Model file for the job. Use its own axes, mm. A direction names the side the tool comes from. Give positions to 0.01 mm unless a question says otherwise; leave off trailing zeros. Order: outer loops, then holes, each group sorted by start corner. A loop starts at its lowest first (then second) coordinate and runs counter-clockwise, first axis right, second up. Notation, with made-up numbers: (14.5, 2.25) -> (55.5, 2.25) arc R12 cw to (55.5, 21.25) -> close; hole circle Ø11 at (33.5, 27.5). An arc over 180 degrees is marked (long way). Use CSV: the item, a comma, the result in double quotes. Start each with the question number.
1. 3-axis set-ups, long thin cutter, end or side, ignore diameter. For faces 5 (the flat face through (0, -18, 15)), 6 (the flat face through (0, -11, -13.675)), 7 (the flat face through (1, 3, 0)): which of +Z, -Z, +X, -X, +Y, -Y reach the whole face in a straight line?
2. Cut at A-A on x = -8.89. List the corners of the cut face in (y, z).
3. Wall check: line 1 (X direction, y = -20, z = -14) (3 decimals); line 2 (Z direction, x = -8.89, y = 1.25); line 3 (X direction, y = -10.5, z = -2) (3 decimals). Give the ranges that are in metal, low to high. Write a range as from..to.
4. Cut at D-D on z = 9.5. List the corners of the cut face in (x, y) (3 decimals), then the cut area to 3 significant figures.
5. Cut at B-B on y = -3.25. List the corners of the cut face in (x, z) (3 decimals), then the cut area to 3 significant figures.
6. Pull direction Z, two halves, no side cores. Call faces 1 (the cylindrical face through (20.85, 1.48, -1.83)), 2 (the flat face through (1, -10, -16.675)), 3 (the flat face through (-39.995, -10, 0)), 4 (the cylindrical face through (-38.85, -9.82, 14.07)): released by +Z, released by -Z, zero draft, split by the parting line, or undercut.
7. Cut at C-C on z = -1. List the corners of the cut face in (x, y) (1 decimal), then the cut area to 3 significant figures.
8. Drop flat-ended pins along their axis: pin 1 (0.9 mm diameter, centred on x = -6, z = 15.5, fed in from -Y); pin 2 (8 mm diameter, centred on x = 8, z = 5, fed in from -Y). Give the stop position or say it passes through.
Autodesk Inventor part; units mm, degrees
ref_plane "YZ Plane" through (0, 0, 0) normal (1, 0, 0) x (0, 1, 0)
ref_plane "XZ Plane" through (0, 0, 0) normal (0, 1, 0) x (-1, 0, 0)
ref_plane "XY Plane" through (0, 0, 0) normal (0, 0, 1) x (1, 0, 0)
sketch "Sketch1" plane through (0, 0, 0) normal (0, 1, 0) x (-1, 0, 0)
  line L0 (39.995, 16.6749) -> (-40.005, 16.6749)
  line L1 (-40.005, 16.6749) -> (-40.005, -16.6751)
  line L2 (-40.005, -16.6751) -> (39.995, -16.6751)
  line L3 (39.995, -16.6751) -> (39.995, 16.6749)
  circle A0 centre (-26.67, -0.0001) radius 6.1
  circle A1 centre (-8.89, -0.0001) radius 6.1
  circle A2 centre (8.89, -0.0001) radius 6.1
  circle A3 centre (26.67, -0.0001) radius 6.1
  point P0 (0, 0)
  dimension "d0" = 33.35
  dimension "d1" = 80
  dimension "d2" = 16.6751
  dimension "d3" = 40.005
  dimension "d4" = 12.2
  dimension "d5" = 13.335
  dimension "d8" = 17.78
extrude "Extrusion1" add sketch "Sketch1" along normal blind 3
sketch "Sketch2" plane through (0, 0, 0) normal (0, -1, 0) x (1, 0, 0)
  circle A0 centre (-26.67, -0.0001) radius 6.1
  circle A1 centre (-8.89, -0.0001) radius 6.1
  circle A2 centre (8.89, -0.0001) radius 6.1
  circle A3 centre (26.67, -0.0001) radius 6.1
  line L0 (-39.995, -16.6751) -> (-39.995, 16.6749)
  line L1 (-39.995, 16.6749) -> (40.005, 16.6749)
  line L2 (40.005, 16.6749) -> (40.005, -16.6751)
  line L3 (40.005, -16.6751) -> (-39.995, -16.6751)
  line L4 (33.899, -13.6749) -> (-33.899, -13.6749)
  line L5 (-33.899, -13.6749) -> (-33.899, 13.6749)
  line L6 (-33.899, 13.6749) -> (33.899, 13.6749)
  line L7 (33.899, 13.6749) -> (33.899, -13.6749)
  line L8 (33.899, -13.6749) -> (-33.899, 13.6749) construction
  line L9 (-33.899, -13.6749) -> (33.899, 13.6749) construction
  point P0 (0, 0)
  dimension "d15" = 6.096
  dimension "d16" = 6.106
  dimension "d17" = 3
  dimension "d18" = 7.229
extrude "Extrusion2" add sketch "Sketch2" along normal blind 23 contours L0 L1 L2 L3
sketch "Sketch4" plane through (-39.995, 3, 16.6749) normal (0, 0, 1) x (1, 0, 0)
  line L0 (80, -26) -> (0, -26)
  line L1 (0, -26) -> (0, 0)
  line L2 (0, 0) -> (80, 0)
  line L3 (80, 0) -> (80, -26)
  line L4 (0, 0) -> (80, 0)
  line L5 (6.096, 0) -> (6.096, -26)
  line L6 (73.894, 0) -> (73.894, -26)
  line L7 (73.894, -3) -> (73.894, -26)
  line L8 (6.096, -21) -> (73.894, -21)
  point P0 (39.995, -3)
  dimension "d21" = 6.096
  dimension "d22" = 6.106
  dimension "d23" = 5
extrude "Extrusion3" cut sketch "Sketch4" against normal blind 23 contours L0 L5 L8 L6
sketch "Sketch5" plane through (0, 3, 0) normal (0, 1, 0) x (1, 0, 0)
  circle A0 centre (-26.67, 0.0001) radius 6.1
  circle A1 centre (-8.89, 0.0001) radius 6.1
  circle A2 centre (8.89, 0.0001) radius 6.1
  circle A3 centre (26.67, 0.0001) radius 6.1
  line L0 (-39.995, -16.6749) -> (-39.995, 16.6751)
  line L1 (-39.995, 16.6751) -> (40.005, 16.6751)
  line L2 (40.005, 16.6751) -> (40.005, -16.6749)
  line L3 (40.005, -16.6749) -> (-39.995, -16.6749)
  line L4 (-33.899, 13.6749) -> (-33.899, -16.6749)
  line L5 (33.899, -13.6749) -> (-33.899, -13.6749)
  line L6 (33.899, 13.6749) -> (-33.899, 13.6749)
  line L7 (33.899, -16.6749) -> (33.899, 13.6749)
  line L8 (-33.67, -12.4999) -> (-19.67, -12.4999)
  line L9 (-19.67, -12.4999) -> (-19.67, 12.5001)
  line L10 (-19.67, 12.5001) -> (-33.67, 12.5001)
  line L11 (-33.67, 12.5001) -> (-33.67, -12.4999)
  line L12 (-33.67, -12.4999) -> (-19.67, 12.5001) construction
  line L13 (-19.67, -12.4999) -> (-33.67, 12.5001) construction
  line L14 (-15.89, -12.4999) -> (-1.89, -12.4999)
  line L15 (-1.89, -12.4999) -> (-1.89, 12.5001)
  line L16 (-1.89, 12.5001) -> (-15.89, 12.5001)
  line L17 (-15.89, 12.5001) -> (-15.89, -12.4999)
  line L18 (1.89, -12.4999) -> (15.89, -12.4999)
  line L19 (15.89, -12.4999) -> (15.89, 12.5001)
  line L20 (15.89, 12.5001) -> (1.89, 12.5001)
  line L21 (1.89, 12.5001) -> (1.89, -12.4999)
  line L22 (19.67, -12.4999) -> (33.67, -12.4999)
  line L23 (33.67, -12.4999) -> (33.67, 12.5001)
  line L24 (33.67, 12.5001) -> (19.67, 12.5001)
  line L25 (19.67, 12.5001) -> (19.67, -12.4999)
  circle A4 centre (-37.455, -14.1349) radius 1.397
  line L26 (0.005, -16.6749) -> (0.005, 16.6751)
  line L27 (-1.89, 0.0001) -> (1.89, 0.0001)
  circle A5 centre (37.465, -14.1349) radius 1.397
  circle A6 centre (-37.455, 14.1351) radius 1.397
  circle A7 centre (37.465, 14.1351) radius 1.397
  point P0 (0, 0)
  dimension "d26" = 13.335
  dimension "d27" = 7.229
  dimension "d28" = 14
  dimension "d29" = 25
  dimension "d30" = 0.229
  dimension "d33" = 17.78
  dimension "d38" = 3.78
  dimension "d39" = 6.325
  dimension "d40" = 2.794
  dimension "d41" = 2.54
  dimension "d44" = 2.54
  dimension "d45" = 2.54
extrude "Extrusion4" cut sketch "Sketch5" against normal blind 50.8 contours A4 | A5 | A6 | A7
properties part number "SwitchPanel"
Verdict:
1,face 5,"+Z, -Y"
1,face 6,"-Y"
1,face 7,"+Z, -Z, +X, -X, +Y"
2,outline,"(-23, -16.68) -> (3, -16.68) -> (3, -6.1) -> (0, -6.1) -> (0, -13.67) -> (-23, -13.67) -> close; (-18, 13.67) -> (0, 13.67) -> (0, 6.1) -> (3, 6.1) -> (3, 16.67) -> (-18, 16.67) -> close"
3,line 1,"-39.995..-38.845, -36.065..36.075, 38.855..40.005"
3,line 2,"-16.68..-6.1, 6.1..16.67"
3,line 3,"-39.995..-33.899, 33.899..40.005"
4,outline,"(-39.995, -23) -> (-33.899, -23) -> (-33.899, 0) -> (33.899, 0) -> (33.899, -23) -> (40.005, -23) -> (40.005, 3) -> (-39.995, 3) -> close"
4,area,"521 mm^2"
5,outline,"(-39.995, -16.675) -> (40.005, -16.675) -> (40.005, 16.675) -> (-39.995, 16.675) -> close; hole circle Ø2.794 at (-37.455, -14.135); hole circle Ø2.794 at (-37.455, 14.135); hole (-33.899, -13.675) -> (33.899, -13.675) -> (33.899, 13.675) -> (-33.899, 13.675) -> close; hole circle Ø2.794 at (37.465, -14.135); hole circle Ø2.794 at (37.465, 14.135)"
5,area,"789 mm^2"
6,face 1,"undercut"
6,face 2,"released by -Z"
6,face 3,"zero draft"
6,face 4,"undercut"
7,outline,"(-40, -23) -> (-33.9, -23) -> (-33.9, 0) -> (-32.7, 0) -> (-32.7, 3) -> (-40, 3) -> close; (-20.7, 0) -> (-14.9, 0) -> (-14.9, 3) -> (-20.7, 3) -> close; (-2.9, 0) -> (2.9, 0) -> (2.9, 3) -> (-2.9, 3) -> close; (14.9, 0) -> (20.7, 0) -> (20.7, 3) -> (14.9, 3) -> close; (32.7, 0) -> (33.9, 0) -> (33.9, -23) -> (40, -23) -> (40, 3) -> (32.7, 3) -> close"
7,area,"376 mm^2"
8,pin 1,"y = -18"
8,pin 2,"y = 0"
